For this review, use the dimensioned drawing (mm, ordinates from the lowest corner) and the shaded views. Coordinates: 2 decimals unless noted, no trailing zeros. Write each loop counter-clockwise with the first axis right and the second up, starting at its lowest first coordinate (ties: lowest second). Pieces come first, ordered by that corner, then holes. Notation, with made-up numbers: (43.25, 53) - (100.25, 53) arc R17 cw to (100.25, 65) - close; hole circle Ø1 at (82.25, 18). An arc over 180 degrees is marked (long way). Answer as a JSON object with one key per item and string values.
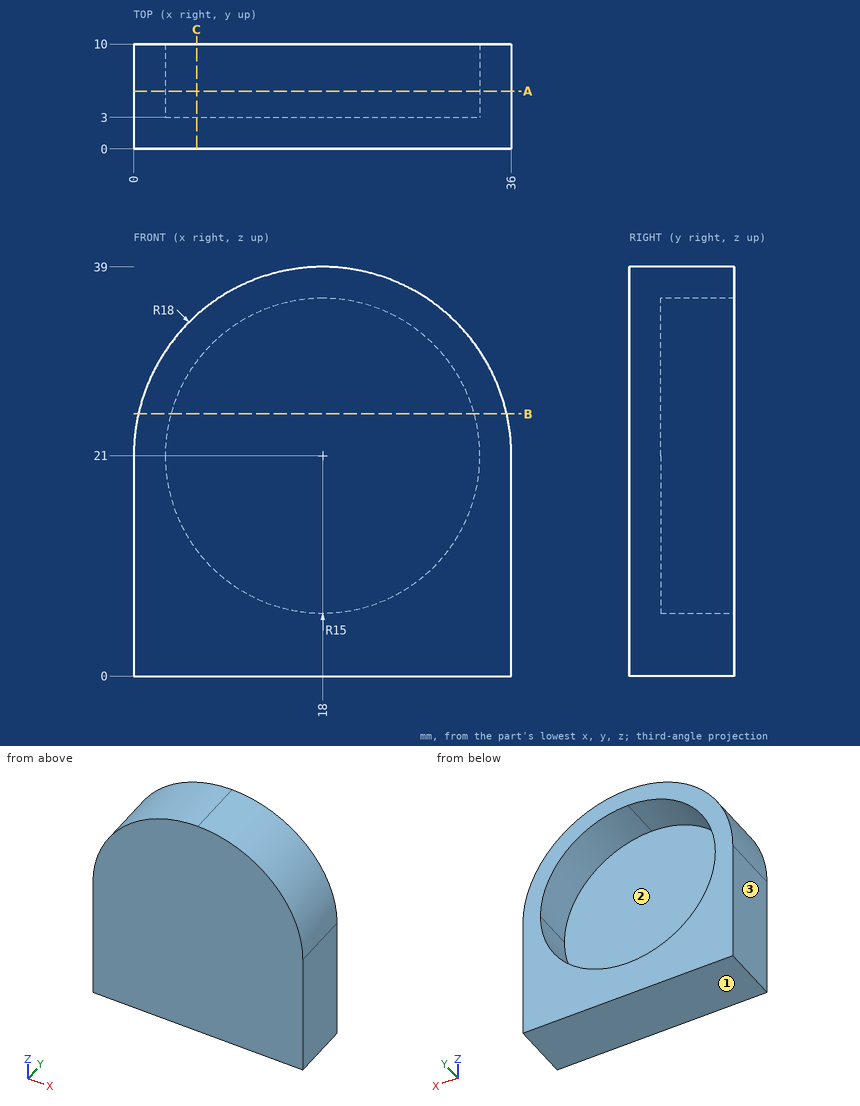
(1) The part is to be moulded in two halves that separate along Z. For the marked faces 1, 2 and 3, say which applies: pulls with the +Z half, pulls with the -Z half, needs draft (parallel to the pull), parting line crosses it, or undercut.
Solved:
{"face 1": "pulls with the -Z half", "face 2": "undercut", "face 3": "needs draft"}
(2) Take a section at A-A, the plane y = 5.5. Write out the cut boundary in (x, z).
Solved:
{"outline": "(0, 0) - (36, 0) - (36, 21) arc R18 ccw to (0, 21) - close; hole (18, 36) arc R15 ccw (long way) to (33, 21) arc R15 ccw to start"}
(3) To check wall thickness, follow line 1 (X direction, y = 5.5, z = 21); line 2 (Y direction, x = 22.5, z = 15); line 3 (X direction, y = 5, z = 18.5). State the ranges of each line that lie inside material, in increasing order. Write a range as from..to.
Solved:
{"line 1": "x = 0..3, 33..36", "line 2": "y = 0..3", "line 3": "x = 0..3.21, 32.79..36"}
(4) Take a section at C-C, the plane x = 6. Write out the cut boundary in (y, z), and give its area (3 significant figures).
Solved:
{"outline": "(0, 0) - (10, 0) - (10, 12) - (3, 12) - (3, 30) - (10, 30) - (10, 34.42) - (0, 34.42) - close", "area": "218 mm^2"}
(5) Take a section at B-B, the plane z = 25. Write out the cut boundary in (x, y).
Solved:
{"outline": "(0.45, 0) - (35.55, 0) - (35.55, 10) - (32.46, 10) - (32.46, 3) - (3.54, 3) - (3.54, 10) - (0.45, 10) - close"}
(6) For pin 1 (2 mm diameter, centred on x = 8.5, z = 11.5, fed in from +Y), flat-tipped, find the tip position at first contact; note if it passes through.
Solved:
{"pin 1": "stops at y = 3"}
